Here's the drawing with two shaded views (mm, measured from the low corner). I have some questions. A direction names the side the tool comes from. Coordinates: 2 decimals unless noted, no trailing zeros. Write each loop counter-clockwise with the first axis right and the second up, starting at its lowest first coordinate (ties: lowest second). Pieces come first, ordered by that corner, then holes. Notation, with made-up numbers: (50, -5.75) -> (60, -5.75) arc R18 ccw to (60, 28.25) -> close; hole circle Ø9 at (-2.5, 14). An arc over 180 degrees is marked (long way). Put each result on its own line as item: value. Start each with the question number.
Item 1: I want a section at C-C, the plane y = 8.75. List the corners of the cut face in (x, z) for me (1 decimal).
Item 2: I want a section at B-B, the plane z = 9.75. List the corners of the cut face in (x, y) for me (1 decimal), then the cut area to 3 significant figures.
Item 3: On a 3-axis mill with a long thin cutter (end or side, diameter ignored), from which of +Z, -Z, +X, -X, +Y, -Y can I reach the whole of each face in a straight line? I mean the marked faces 1 and 2. Say none if no direction works.
Item 4: For pin 1 (6 mm diameter, centred on y = 2, z = 1.5, fed in from -X) (3 decimals); pin 2 (4 mm diameter, centred on x = 19.5, z = 10.5, fed in from -Y); pin 3 (5 mm diameter, centred on x = 26, y = 8.5, fed in from +Z), each with a flat end and sliding along its axis, tell me the tip position at first contact or that it passes through.
Item 5: I need wall thicknesses on line 1 (X direction, y = 5.5, z = 10.5) (1 decimal); line 2 (Y direction, x = 25, z = 9); line 3 (Z direction, x = 29.5, y = 5) (1 decimal). Which ranges of each line are inside material? Lowest first, please. Write a range as [from, to].
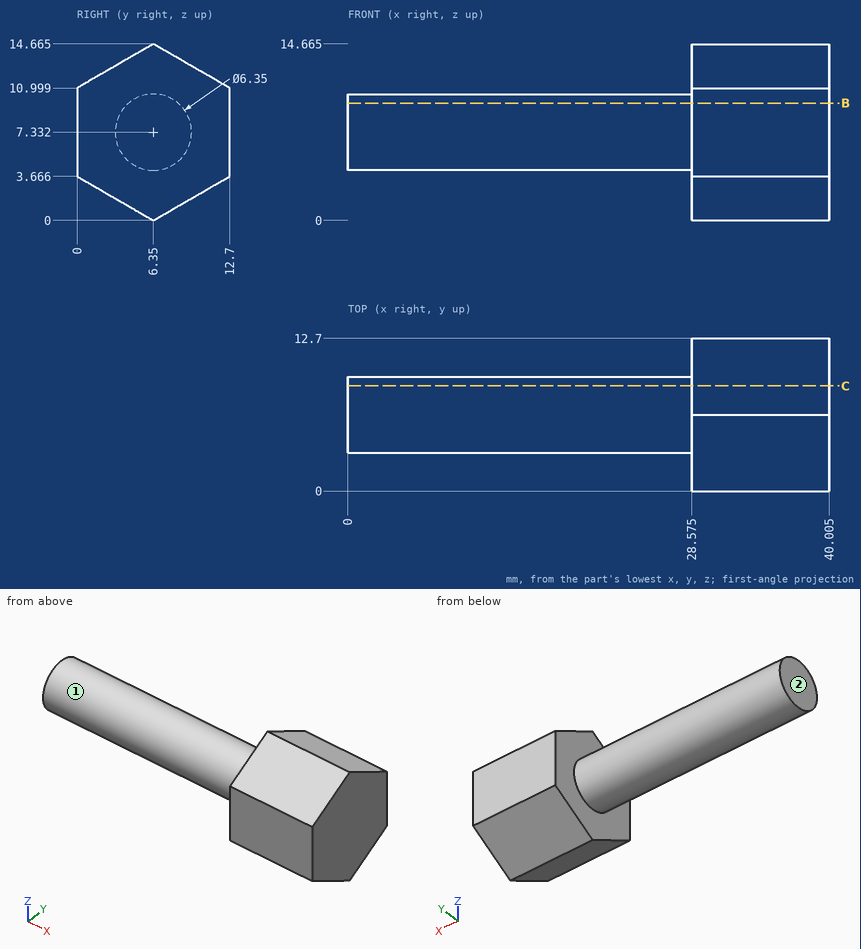
Calculated:
1. outline: (0, 5.3) -> (28.6, 5.3) -> (28.6, 1.4) -> (40, 1.4) -> (40, 13.3) -> (28.6, 13.3) -> (28.6, 9.4) -> (0, 9.4) -> close
2. outline: (0, 4.3) -> (28.6, 4.3) -> (28.6, 0) -> (40, 0) -> (40, 12.7) -> (28.6, 12.7) -> (28.6, 8.4) -> (0, 8.4) -> close
2. area: 263 mm2
3. face 1: -X
3. face 2: +Z, -Z, -X, +Y, -Y
4. pin 1: stops at x = 28.575
4. pin 2: stops at y = 3.4
4. pin 3: stops at z = 10.51
5. line 1: x = [28.6, 40]
5. line 2: y = [3.65, 9.05]
5. line 3: z = [0.8, 13.9]
